CAD build for the part. Positions are in the model's coordinates, mm. A direction names the side the tool comes from. Give positions to 0.01 mm unless a question says otherwise; leave off trailing zeros. Write each loop counter-clockwise with the first axis right and the second up, starting at its lowest first coordinate (ties: lowest second). Pieces come first, ordered by that corner, then holes. Notation, with made-up numbers: (8.5, 68.25) - (65.5, 68.25) arc R25 ccw to (65.5, 82.25) - close; hole circle Ø4 at (58.25, 39). An arc over 180 degrees is marked (long way). Answer as a JSON object with one key per item and string values.
from build123d import *

# Parameters (mm, degrees)
BOSS_EXTRUDE1_DEPTH                     = 10
CBORE_FOR_M5_HEX_HEAD_BOLT1_D           = 5.3
CBORE_FOR_M5_HEX_HEAD_BOLT1_CBORE_D     = 12.24
CBORE_FOR_M5_HEX_HEAD_BOLT1_CBORE_DEPTH = 3.58
SKETCH7_R                               = 10
BOSS_EXTRUDE2_DEPTH                     = 100


with BuildPart() as part:
    # Sketch1 → Boss-Extrude1 (new body)
    with BuildSketch(Plane(origin=(0, 0, 0), x_dir=(1, 0, 0), z_dir=(0, 1, 0))):
        with BuildLine():
            Line((-20, -30), (20, -30))
            ThreePointArc((20, -30), (27.071067812, -27.071067812), (30, -20))
            Line((30, -20), (30, 20))
            ThreePointArc((30, 20), (27.071067812, 27.071067812), (20, 30))
            Line((20, 30), (-20, 30))
            ThreePointArc((-20, 30), (-27.071067812, 27.071067812), (-30, 20))
            Line((-30, 20), (-30, -20))
            ThreePointArc((-30, -20), (-27.071067812, -27.071067812), (-20, -30))
        make_face()
    extrude(amount=BOSS_EXTRUDE1_DEPTH)

    # CBORE for M5 Hex Head Bolt1 (through all)
    with Locations(Plane(origin=(0, 10, 0), x_dir=(1, 0, 0), z_dir=(0, 1, 0))):
        with Locations((-20, -20), (-20, 20), (20, 20), (20, -20)):
            CounterBoreHole(CBORE_FOR_M5_HEX_HEAD_BOLT1_D / 2, CBORE_FOR_M5_HEX_HEAD_BOLT1_CBORE_D / 2, CBORE_FOR_M5_HEX_HEAD_BOLT1_CBORE_DEPTH)

    # Sketch7 → Boss-Extrude2 (add)
    with BuildSketch(Plane(origin=(0, 10, 0), x_dir=(1, 0, 0), z_dir=(0, 1, 0))):
        with Locations(Location((0, 0, 0), (0, 0, 90))):
            Circle(SKETCH7_R)
    extrude(amount=BOSS_EXTRUDE2_DEPTH)


solid = part.part
Item 1: Mould opens along X. For faces 3 (the cylindrical face through (-22.528, 3.165, 19.204)), 4 (the cylindrical face through (26.99, 4.93, 27.15)), 5 (the cylindrical face through (9.76, 59.3, 2.17)), 6 (the flat face through (0, 5, -30)) say: +X half, -X half, draft (parallel to the pull), parting line (faces both ways), or undercut.
Entries:
{"face 3": "undercut", "face 4": "+X half", "face 5": "parting line", "face 6": "draft"}
Item 2: Cut at B-B (z = 8). Give the cut face in (x, y).
Entries:
{"outline": "(-30, 0) - (30, 0) - (30, 10) - (6, 10) - (6, 110) - (-6, 110) - (-6, 10) - (-30, 10) - close"}
Item 3: Probe line 1 (Z direction, x = -20, y = 8.8); line 2 (X direction, y = 2, z = 20). List the from-to ranges inside material, lowest first. Write a range as from..to.
Entries:
{"line 1": "-30..-26.12, -13.88..13.88, 26.12..30", "line 2": "-30..-22.65, -17.35..17.35, 22.65..30"}
Item 4: Cut at C-C (z = 21.5). Give the cut face in (x, y), and give its area (3 significant figures).
Entries:
{"outline": "(-29.89, 0) - (-22.18, 0) - (-22.18, 6.42) - (-25.93, 6.42) - (-25.93, 10) - (-29.89, 10) - close; (-17.82, 0) - (17.82, 0) - (17.82, 6.42) - (14.07, 6.42) - (14.07, 10) - (-14.07, 10) - (-14.07, 6.42) - (-17.82, 6.42) - close; (22.18, 0) - (29.89, 0) - (29.89, 10) - (25.93, 10) - (25.93, 6.42) - (22.18, 6.42) - close", "area": "457 mm2"}
Item 5: Cut at A-A (x = 0). Give the cut face in (y, z), and give its area (3 significant figures).
Entries:
{"outline": "(0, -30) - (10, -30) - (10, -10) - (110, -10) - (110, 10) - (10, 10) - (10, 30) - (0, 30) - close", "area": "2,600 mm2"}
Item 6: Cut at D-D (y = 73). Give the cut face in (x, z).
Entries:
{"outline": "circle Ø20 at (0, 0)"}
Item 7: Which spindle directions (+Z, -Z, +X, -X, +Y, -Y) get a long thin tool onto all of the face, cutting with end or side? Do faces 1 (the cylindrical face through (17.472, 3.165, -20.796)), 2 (the cylindrical face through (-16.71, 8.24, 14.84)). Say none if no direction does.
Entries:
{"face 1": "+Y, -Y", "face 2": "+Y"}
Item 8: Flat gauge pins, fed straight in: P1, Ø6, axis at x = -21.5, z = 23, coming from the +Y side; P2, Ø10, axis at x = 20, z = -20, coming from the +Y side; P3, Ø1.5, axis at x = -20.5, z = 16, coming from the -Y side; P4, Ø5, axis at y = 34.5, z = 0, coming from the -X side. Where does each tip first touch, or does it go through?
Entries:
{"P1": "y = 10", "P2": "y = 6.42", "P3": "y = 0", "P4": "x = -10"}
